Input: dimensioned drawing with shaded views. Units: mm. Origin: part minimum x, y, z. A direction names the side the tool comes from. Coordinates: 2 decimals unless noted, no trailing zeros. Order: outer loops, then holes, each group sorted by start corner. A loop starts at its lowest first (then second) coordinate and runs counter-clockwise, first axis right, second up. Notation, with made-up numbers: (-8.5, -17) - (22.5, -17) arc R27 cw to (22.5, 17) - close; hole circle Ø10 at (83, -11). An arc over 180 degrees is marked (long way). Use one line per item in the form item = value. Start each with the question number.
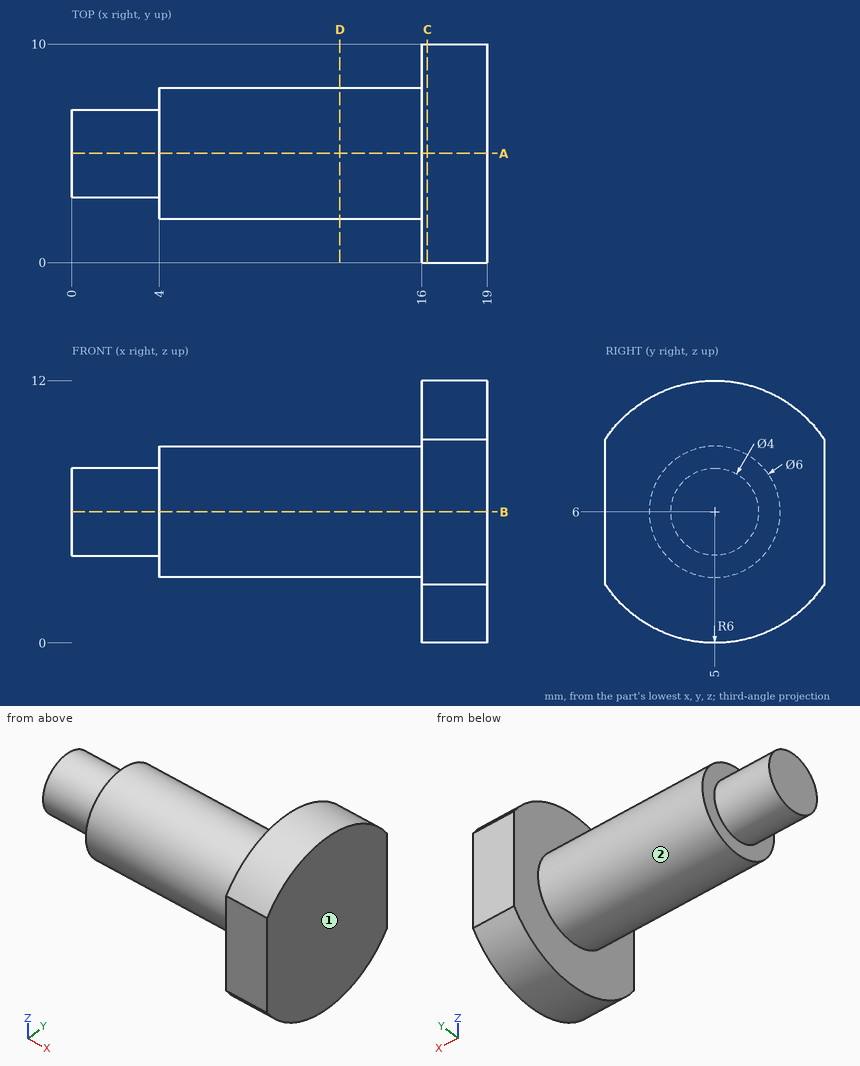
(1) Cut plane B-B on z = 6. Return the cut outline in (x, y), plus the area to 3 significant figures.
(2) Cut plane D-D on x = 12.25. Return the cut outline in (y, z).
(3) Cut plane A-A on y = 5. Return the cut outline in (x, z).
(4) Cut plane C-C on x = 16.25. Return the cut outline in (y, z), plus the area to 3 significant figures.
(5) Contact query for flat-ended pins moving along their axis: pin 1 Ø6 at (x, z) = (11, 9.5) entering from -Y; pin 2 Ø1 at (x, y) = (16.5, 8) entering from -Z; pin 3 Ø5 at (y, z) = (8.5, 5) entering from -X. Output: stop coordinate, or through.
(6) Material intervals for L1, parallel to X at y = 7, z = 3.25; L2, parallel to Z at x = 13.25, y = 6.25; L3, parallel to Z at x = 17.25, y = 1.75, sorted ascending. Write a range as from..to.
(7) Set-up query: the marked faces 1 and 2. Return all of +Z, -Z, +X, -X, +Y, -Y with unobstructed straight access to the full face (end or side cutting, diameter ignored); none if empty.
Check sheet entries:
q1.outline = (0, 3) - (4, 3) - (4, 2) - (16, 2) - (16, 0) - (19, 0) - (19, 10) - (16, 10) - (16, 8) - (4, 8) - (4, 7) - (0, 7) - close
q1.area = 118 mm^2
q2.outline = circle Ø6 at (5, 6)
q3.outline = (0, 4) - (4, 4) - (4, 3) - (16, 3) - (16, 0) - (19, 0) - (19, 12) - (16, 12) - (16, 9) - (4, 9) - (4, 8) - (0, 8) - close
q4.outline = (0, 2.68) arc R6 ccw to (10, 2.68) - (10, 9.32) arc R6 ccw to (0, 9.32) - close
q4.area = 104 mm^2
q5.pin_1 = 2.04
q5.pin_2 = 0.55
q5.pin_3 = 0
q6.L1 = 16..19
q6.L2 = 3.27..8.73
q6.L3 = 0.96..11.04
q7.face_1 = +Z, -Z, +X, +Y, -Y
q7.face_2 = -X
